Model file for the job. Use its own axes, mm. A direction names the side the tool comes from. Coordinates: 2 decimals unless noted, no trailing zeros. Order: outer loops, then holes, each group sorted by start corner. A loop starts at its lowest first (then second) coordinate and runs counter-clockwise, first axis right, second up. Notation, with made-up numbers: (-12.75, 36) -> (15.25, 36) arc R17 ccw to (15.25, 62) -> close; hole circle Ø2 at (42, 18.5). An arc over 180 degrees is marked (long way). Use CSV: the item, a comma, the result in double quotes. Start each with the question number.
(1) Cut at A-A on z = 0. Write the cut outline in (x, y), plus the area to 3 significant figures.
(2) Cut at C-C on x = -38. Write the cut outline in (y, z).
(3) Tool access for faces 1 (the flat face through (17.5, 16.4, 19.1)), 2 (the cylindrical face through (0.25, 31.24, -6.94)), 3 (the cylindrical face through (-23.662, 7.509, 23.846)): list every direction of +Z, -Z, +X, -X, +Y, -Y with a clear straight run to the whole face (end or side of a thin tool).
(4) Probe L1, parallel to X at y = 19, z = -21.5; L2, parallel to X at y = 13.5, z = -17.5; L3, parallel to Y at x = 2, z = -1. List the from-to ranges inside material, lowest first.
(5) Cut at D-D on y = -22. Write the cut outline in (x, z), plus the area to 3 significant figures.
(6) Pin check, flat tips, straight feed: pin 1 Ø2 at (y, z) = (-19.5, -4) entering from -X; pin 2 Ø10 at (y, z) = (4.5, 16) entering from -X; pin 3 Ø5 at (y, z) = (21.5, 8.5) entering from +X; pin 4 Ø4 at (x, z) = (18, 22.5) entering from +Y. Stop position of each tip, or through.
```python
from build123d import *

# Parameters (mm, degrees)
F0_W = 100
F0_H = 15
F2_W = 60
F2_H = 25
F4_W = 35
F4_H = 32


with BuildPart() as f1:
    # F0 (on Front) → F1 (revolve)
    with BuildSketch(Plane.XZ):
        with Locations((0, 7.5)):
            Rectangle(F0_W, F0_H)
    revolve(axis=Axis((-0.244819, 0, 0), (1, 0, 0)))

    # F2 (on Front) → F3 (revolve)
    with BuildSketch(Plane.XZ):
        with Locations((0, 12.5)):
            Rectangle(F2_W, F2_H)
    revolve(axis=Axis((16.772865, 0, 0), (-1, 0, 0)))

    # F4 (on Front) → F5 (revolve)
    with BuildSketch(Plane.XZ):
        with Locations((0, 16)):
            Rectangle(F4_W, F4_H)
    revolve(axis=Axis((8.252203, 0, 0), (1, 0, 0)))


solid = f1.part
```
Outcome:
1,outline,"(-50, -15) -> (-30, -15) -> (-30, -25) -> (-17.5, -25) -> (-17.5, -32) -> (17.5, -32) -> (17.5, -25) -> (30, -25) -> (30, -15) -> (50, -15) -> (50, 15) -> (30, 15) -> (30, 25) -> (17.5, 25) -> (17.5, 32) -> (-17.5, 32) -> (-17.5, 25) -> (-30, 25) -> (-30, 15) -> (-50, 15) -> close"
1,area,"4,690 mm2"
2,outline,"circle Ø30 at (0, 0)"
3,face 1,"+X"
3,face 2,"+X, -X"
3,face 3,"-X"
4,L1,"-17.5 to 17.5"
4,L2,"-30 to 30"
4,L3,"-31.98 to 31.98"
5,outline,"(-30, -11.87) -> (-17.5, -11.87) -> (-17.5, -23.24) -> (17.5, -23.24) -> (17.5, -11.87) -> (30, -11.87) -> (30, 11.87) -> (17.5, 11.87) -> (17.5, 23.24) -> (-17.5, 23.24) -> (-17.5, 11.87) -> (-30, 11.87) -> close"
5,area,"2,220 mm2"
6,pin 1,"x = -30"
6,pin 2,"x = -50"
6,pin 3,"x = 30"
6,pin 4,"y = 24.52"
